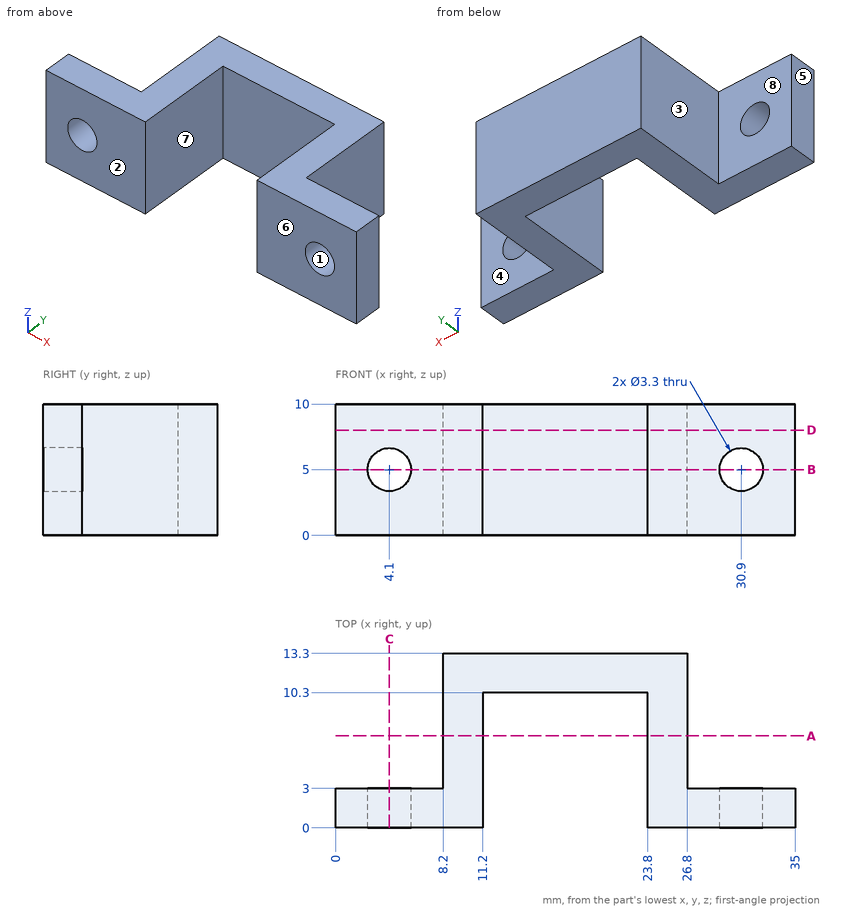
Check sheet for the drawn part. Datum: minimum x, y, z corner. Units: mm. A direction names the side the tool comes from. Round coordinates to 2 decimals unless told otherwise and drop trailing zeros. Order: outer loops, then holes, each group sorted by start corner. A loop starts at its lowest first (then second) coordinate and runs counter-clockwise, first axis right, second up. Notation, with made-up numbers: (8, 33.25) -> (49, 33.25) arc R33 ccw to (49, 64.25) -> close; hole circle Ø3 at (-25, 75). An arc over 180 degrees is marked (long way). Use CSV: the item, a comma, the result in double quotes.
(1) Depth check by flat-ended pin: pin 1 (4 mm diameter, centred on x = 30.5, z = 2.5, fed in from +Y); pin 2 (3 mm diameter, centred on x = 28.5, y = 11, fed in from -Z); pin 3 (1.5 mm diameter, centred on x = 20, z = 1.5, fed in from -Y); pin 4 (2 mm diameter, centred on y = 11.5, z = 3.5, fed in from -X). Enter the tip coordinate at first touch or a pass-through.
Worked out:
pin 1,"y = 3"
pin 2,"through"
pin 3,"y = 10.3"
pin 4,"x = 8.2"
(2) Draft check along X on the marked faces 1, 2 and 3. Enter one of: pulls with the +X half, pulls with the -X half, needs draft (parallel to the pull), parting line crosses it, or undercut.
Worked out:
face 1,"undercut"
face 2,"needs draft"
face 3,"pulls with the -X half"
(3) Cross-section at C-C (x = 4.1). Record the boundary of the cut face in (y, z), and give its area (3 significant figures).
Worked out:
outline,"(0, 0) -> (3, 0) -> (3, 3.35) -> (0, 3.35) -> close; (0, 6.65) -> (3, 6.65) -> (3, 10) -> (0, 10) -> close"
area,"20.1 mm²"
(4) Cross-section at B-B (z = 5). Record the boundary of the cut face in (x, y), and give its area (3 significant figures).
Worked out:
outline,"(0, 0) -> (2.45, 0) -> (2.45, 3) -> (0, 3) -> close; (5.75, 0) -> (11.2, 0) -> (11.2, 10.3) -> (23.8, 10.3) -> (23.8, 0) -> (29.25, 0) -> (29.25, 3) -> (26.8, 3) -> (26.8, 13.3) -> (8.2, 13.3) -> (8.2, 3) -> (5.75, 3) -> close; (32.55, 0) -> (35, 0) -> (35, 3) -> (32.55, 3) -> close"
area,"147 mm²"
(5) Material ranges on line 1 along X through (y, z) = (2.45, 5); line 2 along X through (y, z) = (6.5, 7.75); line 3 along X through (y, z) = (2.25, 1.25), recorded low to high. Write a range as from..to.
Worked out:
line 1,"0..2.45, 5.75..11.2, 23.8..29.25, 32.55..35"
line 2,"8.2..11.2, 23.8..26.8"
line 3,"0..11.2, 23.8..35"
(6) Cross-section at A-A (y = 7). Record the boundary of the cut face in (x, z).
Worked out:
outline,"(8.2, 0) -> (11.2, 0) -> (11.2, 10) -> (8.2, 10) -> close; (23.8, 0) -> (26.8, 0) -> (26.8, 10) -> (23.8, 10) -> close"
(7) Tool access check on the marked faces 4, 5, 6, 7 and 8. Record the directions out of +Z, -Z, +X, -X, +Y, -Y that give a thin tool (end or side, any length) a straight path to the whole face; none if there is none.
Worked out:
face 4,"+Z, -Z, +X, +Y"
face 5,"+Z, -Z, -X, +Y, -Y"
face 6,"+Z, -Z, +X, -X, -Y"
face 7,"+Z, -Z, -Y"
face 8,"+Z, -Z, -X, +Y"
(8) Cross-section at D-D (z = 8). Record the boundary of the cut face in (x, y), and give its area (3 significant figures).
Worked out:
outline,"(0, 0) -> (11.2, 0) -> (11.2, 10.3) -> (23.8, 10.3) -> (23.8, 0) -> (35, 0) -> (35, 3) -> (26.8, 3) -> (26.8, 13.3) -> (8.2, 13.3) -> (8.2, 3) -> (0, 3) -> close"
area,"167 mm²"
